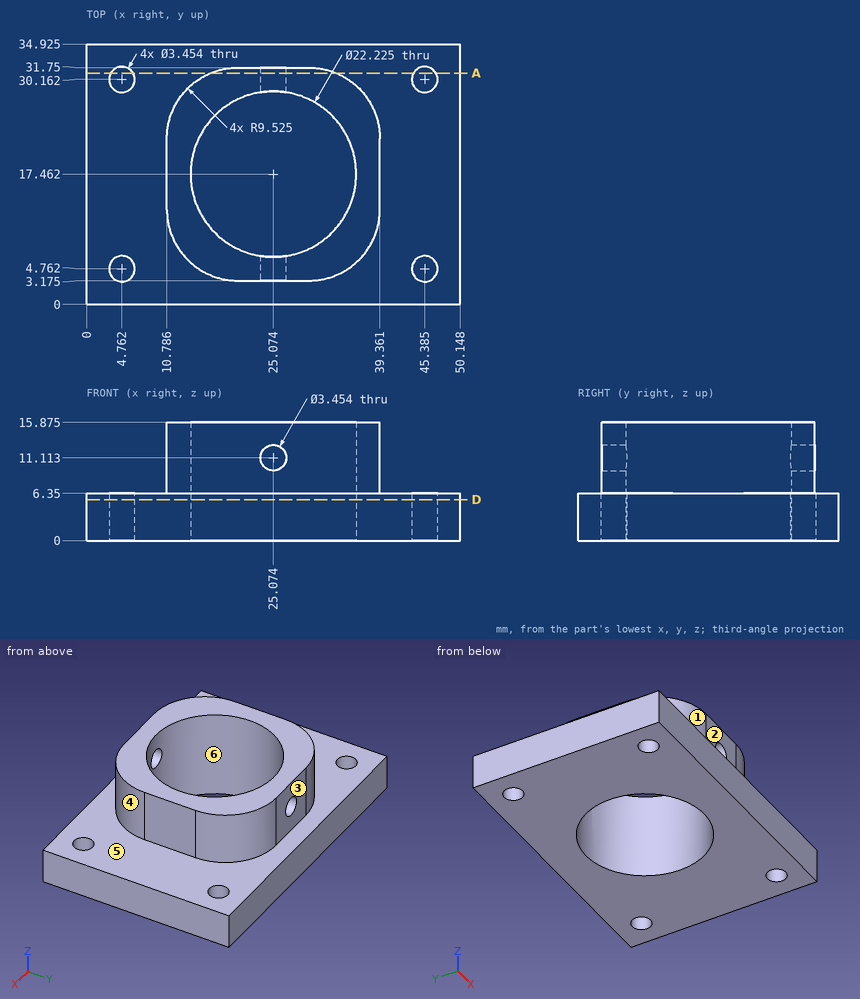
Check sheet for the drawn part. Datum: minimum x, y, z corner. Units: mm. A direction names the side the tool comes from. Coordinates: 2 decimals unless noted, no trailing zeros. Loops run counter-clockwise (first coordinate to the right, second up) from the corner with the lowest first, then second, coordinate; pieces in that order, holes last. Notation, with made-up numbers: (62.5, -38) - (83.5, -38) arc R28 ccw to (83.5, -19) - close; hole circle Ø9 at (10, 35). An arc over 180 degrees is marked (long way). Put each result on its own line as item: value.
Item 1: Gauge pin test, flat ends, axial feed: pin 1 Ø4 at (y, z) = (18.5, 11.5) entering from -X; pin 2 Ø4.5 at (x, y) = (45.39, 30.16) entering from +Z; pin 3 Ø3 at (x, z) = (25.5, 10.5) entering from -Y (1 decimal). Record the tip position at first contact, or that the pin passes through.
Conclusion:
pin 1: stops at x = 10.79
pin 2: stops at z = 6.35
pin 3: stops at y = 3.2
Item 2: Section check D-D (z = 5.5). Enter the section's corners in (x, y) (1 decimal).
Conclusion:
outline: (0, 0) - (50.1, 0) - (50.1, 34.9) - (0, 34.9) - close; hole circle Ø3.5 at (4.8, 4.8); hole circle Ø3.5 at (4.8, 30.2); hole circle Ø22.2 at (25.1, 17.5); hole circle Ø3.5 at (45.4, 4.8); hole circle Ø3.5 at (45.4, 30.2)
Item 3: Scan lines: line 1 along Z through (x, y) = (25, 6) (1 decimal); line 2 along Z through (x, y) = (48.5, 19); line 3 along Y through (x, z) = (35, 8) (1 decimal). Record each from-to range of solid material in increasing order.
Conclusion:
line 1: z = 0 to 9.4, 12.8 to 15.9
line 2: z = 0 to 6.35
line 3: y = 4.7 to 12.5, 22.5 to 30.2
Item 4: Section check A-A (y = 31). Give the number of separate pieces and of enclosed holes in the cut face, then the cut area to 3 significant figures.
Conclusion:
separate pieces: 3
enclosed holes: 1
area: 432 mm2
Item 5: Draft check along Y on the marked faces 4, 5 and 6. Enter one of: pulls with the +Y half, pulls with the -Y half, needs draft (parallel to the pull), parting line crosses it, or undercut.
Conclusion:
face 4: pulls with the -Y half
face 5: needs draft
face 6: undercut
Item 6: Set-up check for the marked faces 1, 2 and 3: record each of +Z, -Z, +X, -X, +Y, -Y from which the full face is reachable in a straight line by a thin tool's end or side.
Conclusion:
face 1: +Z, -X, -Y
face 2: +Z, +X, -X, -Y
face 3: +Z, +X, -X, +Y
